Drawing for the job (mm, zero at the part's lowest x, y, z). Coordinates: 2 decimals unless noted, no trailing zeros. Loops run counter-clockwise (first coordinate to the right, second up) from the corner with the lowest first, then second, coordinate; pieces in that order, holes last.
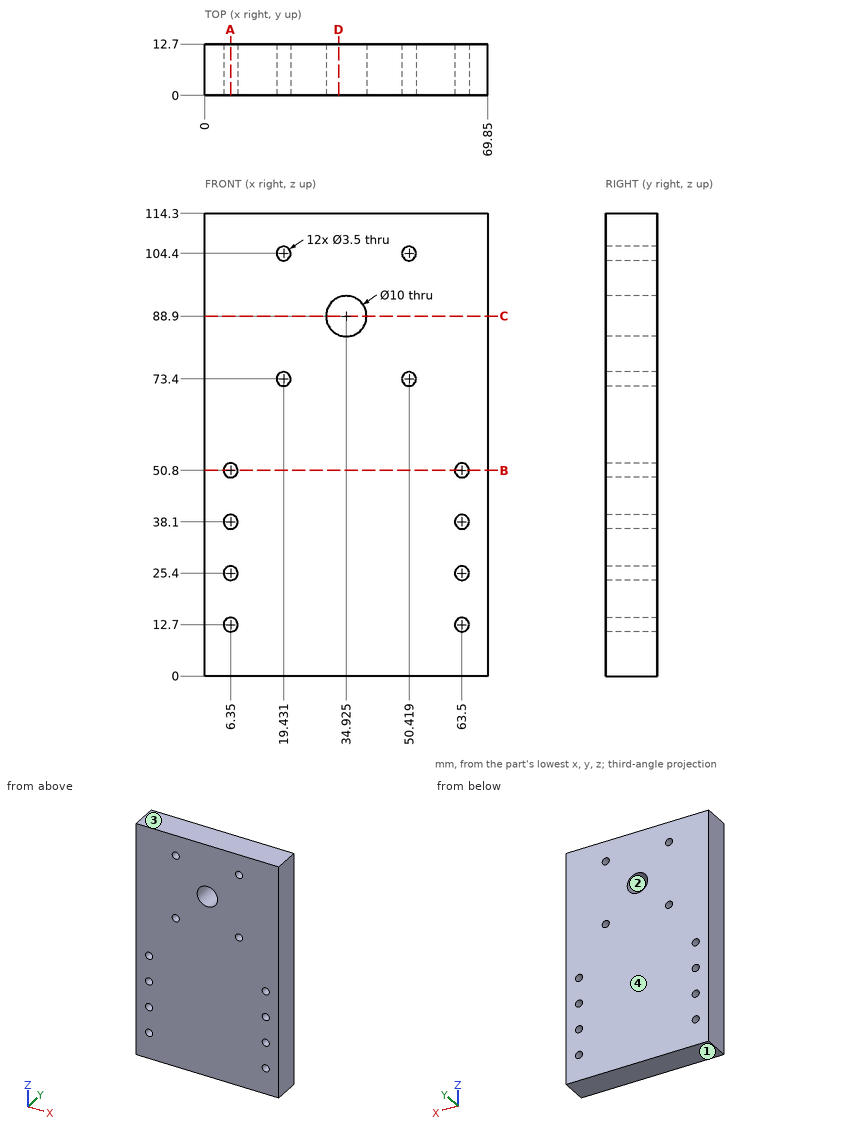
Q1. Drop a flat-ended pin along its axis: P1, Ø4.5, axis at x = 6.35, z = 25.4, coming from the -Y side. Give the stop position or say it passes through.
Q2. Saw through at A-A (x = 6.35). List the corners of the cut face in (y, z).
Q3. Saw through at B-B (z = 50.8). List the corners of the cut face in (x, y), plus the area to 3 significant figures.
Q4. Mould opens along Z. For the marked faces 1, 2, 3 and 4 say: released by +Z, released by -Z, zero draft, split by the parting line, or undercut.
Q5. Saw through at C-C (z = 88.9). List the corners of the cut face in (x, y) (3 decimals), plus the area to 3 significant figures.
Q6. Probe line 1 (X direction, y = 5, z = 25.4); line 2 (X direction, y = 5.75, z = 14); line 3 (Z direction, x = 6.35, y = 5). List the from-to ranges inside material, lowest first.
Q7. Saw through at D-D (x = 33). List the corners of the cut face in (y, z).
Checked values:
1. P1: stops at y = 0
2. outline: (0, 0) - (12.7, 0) - (12.7, 10.95) - (0, 10.95) - close; (0, 14.45) - (12.7, 14.45) - (12.7, 23.65) - (0, 23.65) - close; (0, 27.15) - (12.7, 27.15) - (12.7, 36.35) - (0, 36.35) - close; (0, 39.85) - (12.7, 39.85) - (12.7, 49.05) - (0, 49.05) - close; (0, 52.55) - (12.7, 52.55) - (12.7, 114.3) - (0, 114.3) - close
3. outline: (0, 0) - (4.6, 0) - (4.6, 12.7) - (0, 12.7) - close; (8.1, 0) - (61.75, 0) - (61.75, 12.7) - (8.1, 12.7) - close; (65.25, 0) - (69.85, 0) - (69.85, 12.7) - (65.25, 12.7) - close
3. area: 798 mm2
4. face 1: released by -Z
4. face 2: undercut
4. face 3: released by +Z
4. face 4: zero draft
5. outline: (0, 0) - (29.925, 0) - (29.925, 12.7) - (0, 12.7) - close; (39.925, 0) - (69.85, 0) - (69.85, 12.7) - (39.925, 12.7) - close
5. area: 760 mm2
6. line 1: x = 0 to 4.6, 8.1 to 61.75, 65.25 to 69.85
6. line 2: x = 0 to 5.18, 7.52 to 62.33, 64.67 to 69.85
6. line 3: z = 0 to 10.95, 14.45 to 23.65, 27.15 to 36.35, 39.85 to 49.05, 52.55 to 114.3
7. outline: (0, 0) - (12.7, 0) - (12.7, 84.29) - (0, 84.29) - close; (0, 93.51) - (12.7, 93.51) - (12.7, 114.3) - (0, 114.3) - close
